Input: dimensioned drawing with shaded views. Units: mm. Origin: part minimum x, y, z. A direction names the side the tool comes from. Coordinates: 2 decimals unless noted, no trailing zeros. Order: outer loops, then holes, each group sorted by start corner. A loop starts at its lowest first (then second) coordinate and runs counter-clockwise, first axis right, second up. Notation, with made-up numbers: (-3, 57.25) - (28, 57.25) arc R29 cw to (28, 85.25) - close; hole circle Ø3 at (68.5, -6). An arc over 180 degrees is marked (long way). Use one line per item in the form item = value. Start each with the question number.
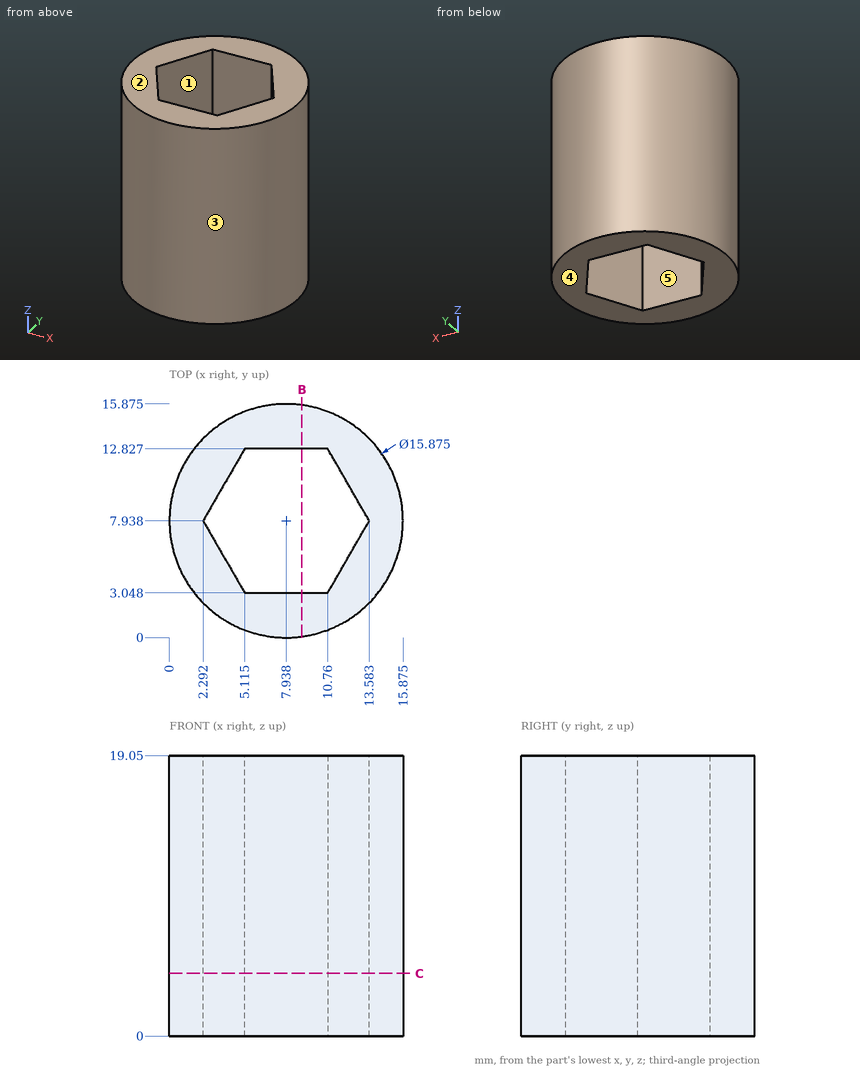
(1) Contact query for flat-ended pins moving along their axis: pin 1 Ø1 at (y, z) = (9, 16.5) entering from +X (1 decimal); pin 2 Ø1 at (x, z) = (12.5, 10.5) entering from -Y; pin 3 Ø5 at (x, z) = (14, 3.5) entering from -Y (1 decimal). Output: stop coordinate, or through.
(2) Cut plane B-B on x = 9. Return the cut outline in (y, z), plus the area to 3 significant figures.
(3) Material intervals for L1, parallel to Y at x = 8.25, z = 7.25; L2, parallel to X at y = 4, z = 9 (1 decimal); L3, parallel to Y at x = 9, z = 12.75, sorted ascending. Write a range as from..to.
(4) Draft query along Y for the marked faces 3, 4 and 5. Return one class per face: released by +Y, released by -Y, zero draft, split by the parting line, or undercut.
(5) Set-up query: the marked faces 1 and 2. Return all of +Z, -Z, +X, -X, +Y, -Y with unobstructed straight access to the full face (end or side cutting, diameter ignored); none if empty.
(6) Cut plane C-C on z = 4.25. Return the cut outline in (x, y) (1 decimal), plus the area to 3 significant figures.
Check sheet entries:
q1.pin_1 = 15.9
q1.pin_2 = 1.12
q1.pin_3 = 0.8
q2.outline = (0.07, 0) - (3.05, 0) - (3.05, 19.05) - (0.07, 19.05) - close; (12.83, 0) - (15.8, 0) - (15.8, 19.05) - (12.83, 19.05) - close
q2.area = 113 mm^2
q3.L1 = 0.01..3.05, 12.83..15.87
q3.L2 = 1..4.6, 11.3..14.8
q3.L3 = 0.07..3.05, 12.83..15.8
q4.face_3 = split by the parting line
q4.face_4 = zero draft
q4.face_5 = undercut
q5.face_1 = +Z, -Z
q5.face_2 = +Z, +X, -X, +Y, -Y
q6.outline = circle Ø15.9 at (7.9, 7.9); hole (2.3, 7.9) - (5.1, 3) - (10.8, 3) - (13.6, 7.9) - (10.8, 12.8) - (5.1, 12.8) - close
q6.area = 115 mm^2
